Can you work these out from the model? Positions are in its coordinate system, mm. A direction names the side the tool comes from. Round coordinates to 2 decimals unless told otherwise and drop trailing zeros. Write each loop counter-clockwise with the first axis right and the second up, starting at its lowest first coordinate (ties: lowest second). Pieces come first, ordered by that corner, then holes. Notation, with made-up numbers: (24.25, 33) -> (74.25, 33) arc R16 ccw to (74.25, 46) -> close; hole circle Ø10 at (22, -7). An arc over 180 degrees is marked (long way). Use CSV: the item, a comma, the result in double quotes.
Autodesk Inventor part; units mm, degrees
ref_plane "YZ Plane" through (0, 0, 0) normal (1, 0, 0) x (0, 1, 0)
ref_plane "XZ Plane" through (0, 0, 0) normal (0, 1, 0) x (-1, 0, 0)
ref_plane "XY Plane" through (0, 0, 0) normal (0, 0, 1) x (1, 0, 0)
sketch "Sketch1" plane through (0, 0, 0) normal (0, 1, 0) x (-1, 0, 0)
  line L0 (0, 0) -> (0, -144)
  line L1 (0, 0) -> (20, 0)
  line L2 (20, 0) -> (20, 3)
  line L3 (20, 3) -> (40, 3)
  line L4 (40, 3) -> (40, 0)
  line L5 (40, 0) -> (60, 0)
  line L6 (60, 0) -> (60, 3)
  line L7 (60, 3) -> (80, 3)
  line L8 (0, -72) -> (20, -72)
  line L9 (0, -144) -> (20, -144)
  line L10 (20, -144) -> (20, -147)
  line L11 (20, -147) -> (40, -147)
  line L12 (40, -147) -> (40, -144)
  line L13 (40, -144) -> (60, -144)
  line L14 (60, -144) -> (60, -147)
  line L15 (60, -147) -> (80, -147)
  line L16 (80, 3) -> (80, -147)
  dimension "d0" = 144
  dimension "d1" = 20
  dimension "d2" = 3
  dimension "d3" = 20
  dimension "d4" = 20
  dimension "d5" = 20
  dimension "d6" = 20
extrude "Extrusion1" add sketch "Sketch1" along normal blind 3
properties part number "base prt 2 N" material "ABS Plastic"
Q1. Suppose I cut it at B-B (x = -12). Write out the boundary of the cut face in (y, z).
Resolved:
outline,"(0, -144) -> (3, -144) -> (3, 0) -> (0, 0) -> close"
Q2. If we mould it in two halves opening along X, with no side actions, what happens to faces 5 (the face through (0, 1, -71)), 6 (the face through (-50, 1, 0)), 7 (the face through (-70, 1, 3)), 8 (the face through (-40, 1, -146))? For each: released by +X, released by -X, zero draft, split by the parting line, or undercut.
Resolved:
face 5,"released by +X"
face 6,"undercut"
face 7,"zero draft"
face 8,"undercut"
Q3. Suppose I cut it at A-A (y = 0.8). Write out the boundary of the cut face in (x, z), and give its area (3 significant figures).
Resolved:
outline,"(-80, -147) -> (-60, -147) -> (-60, -144) -> (-40, -144) -> (-40, -147) -> (-20, -147) -> (-20, -144) -> (0, -144) -> (0, 0) -> (-20, 0) -> (-20, 3) -> (-40, 3) -> (-40, 0) -> (-60, 0) -> (-60, 3) -> (-80, 3) -> close"
area,"11,800 mm^2"
Q4. Please list where this line runs through material, in increasing order: probe 1 along Z at (x, y) = (-12, 0.2).
Resolved:
probe 1,"z = -144 to 0"
Q5. On a 3-axis mill with a long thin cutter (end or side, diameter ignored), from which of +Z, -Z, +X, -X, +Y, -Y can I reach the whole of each face in a straight line? I mean faces 1 (the face through (-20, 1, -145)), 2 (the face through (-50, 1, -144)), 3 (the face through (-60, 1, 1)), 4 (the face through (-10, 1, 0)). Say none if no direction works.
Resolved:
face 1,"-Z, +X, +Y, -Y"
face 2,"-Z, +Y, -Y"
face 3,"+Z, +Y, -Y"
face 4,"+Z, +X, +Y, -Y"
Q6. Will these pins go through, and if not, where does the flat tip stop? P1, Ø0.9, axis at x = -9.5, y = 2, coming from the -Z side; P2, Ø1.5, axis at y = 1, z = 1.5, coming from the +X side; P3, Ø0.9, axis at x = -46, y = 1, coming from the +Z side.
Resolved:
P1,"stops at z = -144"
P2,"stops at x = -20"
P3,"stops at z = 0"
